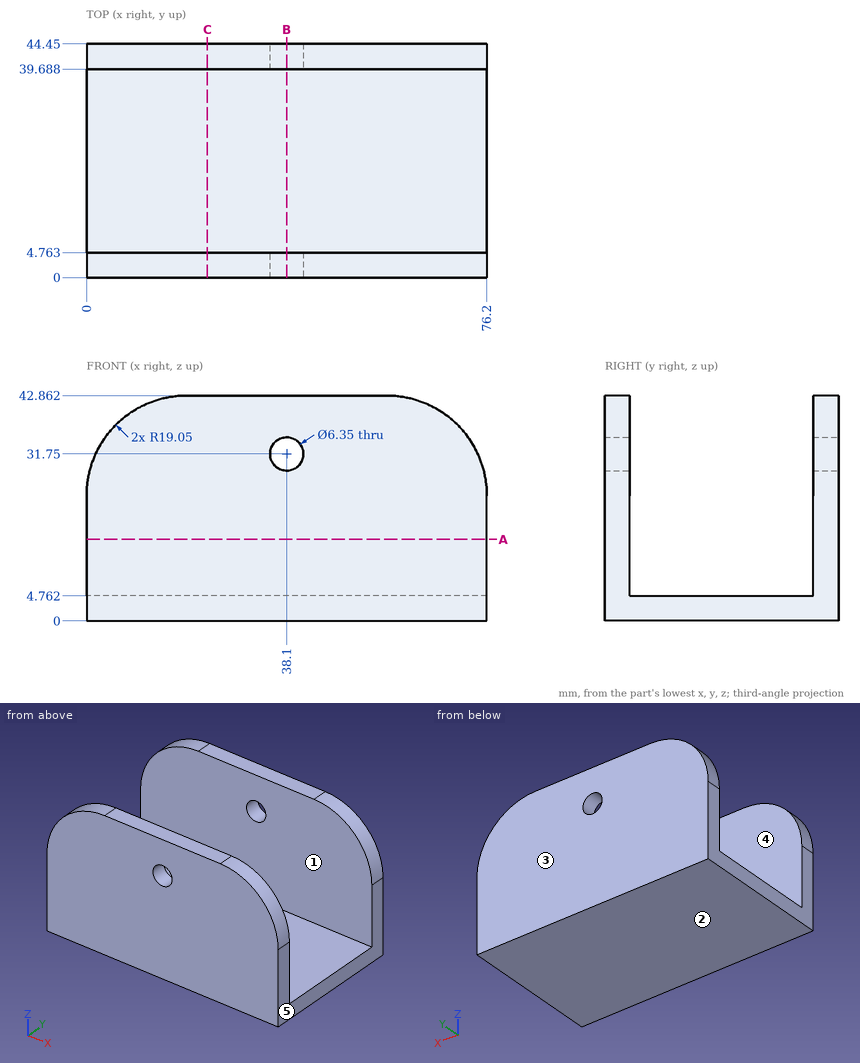
The figure shows three views and two pictorial views of one solid part (mm, origin at its lowest corner). Answer the questions. A direction names the side the tool comes from. Round coordinates to 2 decimals unless told otherwise and drop trailing zeros. Write each loop counter-clockwise with the first axis right and the second up, starting at its lowest first coordinate (ties: lowest second). Pieces come first, ordered by that corner, then holes. Notation, with made-up numbers: (35, 63.5) - (85, 63.5) arc R10 cw to (85, 80.5) - close; hole circle Ø1 at (22.5, 69). An arc over 180 degrees is marked (long way). Use one line per item in the form item = value. Start each with the question number.
Item 1: A cutting plane is placed at A-A (z = 15.5). Write down the section's boundary in (x, y).
Item 2: Flat-ended cylindrical pins translate along their axes: pin 1 Ø2 at (x, y) = (46, 38) entering from -Z; pin 2 Ø3 at (y, z) = (39, 26) entering from +X; pin 3 Ø10.5 at (x, y) = (46, 19.5) entering from +Z. Find the tip coordinate at first contact, or state that the pin passes through.
Item 3: Determine the mould class of the marked faces 3, 4 and 5 for opening direction Y: +Y half, -Y half, draft (parallel to the pull), parting line (faces both ways), or undercut.
Item 4: A tool of negligible diameter and unlimited length cuts with its end or side. For the marked faces 1 and 2, from which of +Z, -Z, +X, -X, +Y, -Y can it reach the whole face along a straight path? Write none if from no direction.
Item 5: A cutting plane is placed at B-B (x = 38.1). Give the number of separate pieces and of enclosed holes in the cut face, plus the area to 3 significant figures.
Item 6: Find the intervals of material crossed by line 1 (Y direction, x = 60, z = 22); line 2 (Z direction, x = 38.1, y = 2.7) (1 decimal); line 3 (Z direction, x = 26, y = 29.5), in increasing order. Write a range as [from, to].
Item 7: A cutting plane is placed at C-C (x = 23). Write down the section's boundary in (y, z).
The answers:
q1.outline = (0, 0) - (76.2, 0) - (76.2, 4.76) - (0, 4.76) - close; (0, 39.69) - (76.2, 39.69) - (76.2, 44.45) - (0, 44.45) - close
q2.pin_1 = 0
q2.pin_2 = 76.18
q2.pin_3 = 4.76
q3.face_3 = +Y half
q3.face_4 = undercut
q3.face_5 = draft
q4.face_1 = +Z, +X, -X
q4.face_2 = -Z, +X, -X, +Y, -Y
q5.separate_pieces = 3
q5.enclosed_holes = 0
q5.area = 514 mm^2
q6.line_1 = [0, 4.76], [39.69, 44.45]
q6.line_2 = [0, 28.6], [34.9, 42.9]
q6.line_3 = [0, 4.76]
q7.outline = (0, 0) - (44.45, 0) - (44.45, 42.86) - (39.69, 42.86) - (39.69, 4.76) - (4.76, 4.76) - (4.76, 42.86) - (0, 42.86) - close
